from build123d import *

# Parameters (mm, degrees)
F0_W     = 75.805991888
F0_H     = 35.9990932047
F1_DEPTH = 25.4
F3_W     = 3.6910921335
F3_H     = 8.858628571
F3_W_2   = 4.4293105602
F3_H_2   = 7.0130825043
F4_DEPTH = 25.4
F5_DEPTH = 25.4
F6_W     = 26.3966843486
F6_H     = 116.8616563082
F7_DEPTH = 25.4
F8_W     = 123.443312943
F8_H     = 25.7022343576
F9_DEPTH = 25.4


with BuildPart() as f1:
    # F0 (on Front) → F1 (new body)
    with BuildSketch(Plane.XZ):
        with Locations((-37.902995944, 57.8962471336)):
            Rectangle(F0_W, F0_H)
    extrude(amount=F1_DEPTH)

    # F3 (on Front) → F4 (join)
    with BuildSketch(Plane.XZ):
        Polygon((-60.510866344, 33.7904244661), (-54.6051189303, 33.7904244661), (-54.6051189303, 33.0522060394), (-60.510866344, 33.0522060394), (-60.510866344, 29.3611101806), (-52.3904636502, 29.3611101806), (-52.3904636502, 38.2197387516), (-60.510866344, 38.2197387516), align=None)
        Polygon((-60.510866344, 33.0522060394), (-60.510866344, 33.7904244661), (-60.510866344, 38.2197387516), (-52.3904636502, 38.2197387516), (-52.3904636502, 59.6280917525), (-75.2752497792, 59.6280917525), (-75.2752497792, -67.7146911621), (-70.845939219, -67.7146911621), (-70.845939219, -74.7277736664), (-52.3904636502, -74.7277736664), (-52.3904636502, 29.3611101806), (-60.510866344, 29.3611101806), align=None)
        with Locations((-50.5449175835, 33.7904244661)):
            Rectangle(F3_W, F3_H)
        with Locations((-73.0605944991, -71.2212324142)):
            Rectangle(F3_W_2, F3_H_2)
        Polygon((-70.845939219, -81.7408561707), (-70.845939219, -74.7277736664), (-75.2752497792, -74.7277736664), (-75.2752497792, -67.7146911621), (-79.7045603395, -67.7146911621), (-79.7045603395, -81.7408561707), align=None)
    extrude(amount=F4_DEPTH)

    # F2 (on Front) → F5 (join)
    with BuildSketch(Plane.XZ):
        Polygon((74.952326715, 40.4343977571), (74.952326715, 75.4998028278), (0, 75.4998028278), (0, 40.4343977571), (25.4916474223, 40.4343977571), align=None)
    extrude(amount=F5_DEPTH)

    # F6 (on Front) → F7 (join)
    with BuildSketch(Plane.XZ):
        with Locations((61.6374202073, -17.1837881207)):
            Rectangle(F6_W, F6_H)
    extrude(amount=F7_DEPTH)

    # F8 (on Front) → F9 (join)
    with BuildSketch(Plane.XZ):
        with Locations((-13.6707611382, -62.0693061501)):
            Rectangle(F8_W, F8_H)
    extrude(amount=F9_DEPTH)


solid = f1.part
Verification items for the finished model (mm, model axes). A direction names the side the tool comes from. Coordinates: 2 decimals unless noted, no trailing zeros. Loops run counter-clockwise (first coordinate to the right, second up) from the corner with the lowest first, then second, coordinate; pieces in that order, holes last. Notation, with made-up numbers: (48.5, -21) -> (53.5, -21) arc R27 ccw to (53.5, 15) -> close; hole circle Ø6 at (47, 47.25). An arc over 180 degrees is marked (long way). Answer as CSV lines item,"result".
1) Depth check by flat-ended pin: pin 1 (1 mm diameter, centred on x = 11, z = -47.5, fed in from +Y); pin 2 (8 mm diameter, centred on x = 46.5, y = -3, fed in from +Z); pin 3 (6 mm diameter, centred on y = -10.5, z = 1, fed in from +X); pin 4 (2 mm diameter, centred on x = -78.5, y = -17.5, fed in from +Z). Enter the tip coordinate at first touch or a pass-through.
Found:
pin 1,"passes through"
pin 2,"stops at z = 75.5"
pin 3,"stops at x = 74.84"
pin 4,"stops at z = -67.71"
2) Thickness scan on L1, parallel to X at y = -17, z = -9; L2, parallel to X at y = -6.25, z = -69.5; L3, parallel to Z at x = -9.5, y = -15.75. Record the ranges inside material, lowest first. Write a range as from..to.
Found:
L1,"x = -75.28..-52.39, 48.44..74.84"
L2,"x = -79.7..48.05, 48.44..74.84"
L3,"z = -74.92..-49.22, 39.9..75.9"
3) Release check for a two-part mould opening along Z. For faces 1 (the flat face through (-75, -13, -81.741)), 2 (the flat face through (-58, -13, 33.052)), 3 (the flat face through (-55, -25.4, -2)), 4 (the flat face through (38, -13, 75.5)) record: +Z half, -Z half, draft (parallel to the pull), parting line (faces both ways), or undercut.
Found:
face 1,"-Z half"
face 2,"undercut"
face 3,"draft"
face 4,"+Z half"
4) Cross-section at D-D, the plane x = 55. Record the cut outline in (y, z), then the cut area to 3 significant figures.
Found:
outline,"(-25.4, -75.61) -> (0, -75.61) -> (0, 75.5) -> (-25.4, 75.5) -> close"
area,"3,840 mm2"
5) Tool access check on faces 5 (the flat face through (-75.392, -13, -59)), 6 (the flat face through (-52.39, -13, -10)), 7 (the flat face through (48.439, -13, -18)). Record the directions out of +Z, -Z, +X, -X, +Y, -Y that give a thin tool (end or side, any length) a straight path to the whole face; none if there is none.
Found:
face 5,"-X, +Y, -Y"
face 6,"+Y, -Y"
face 7,"-Z, +Y, -Y"
6) Cross-section at C-C, the plane z = 6. Record the cut outline in (x, y), then the cut area to 3 significant figures.
Found:
outline,"(-75.28, -25.4) -> (-52.39, -25.4) -> (-52.39, 0) -> (-75.28, 0) -> close; (48.44, -25.4) -> (74.84, -25.4) -> (74.84, 0) -> (48.44, 0) -> close"
area,"1,250 mm2"
7) Cross-section at A-A, the plane x = 17.5. Record the cut outline in (y, z), then the cut area to 3 significant figures.
Found:
outline,"(-25.4, -74.92) -> (0, -74.92) -> (0, -49.22) -> (-25.4, -49.22) -> close; (-25.4, 40.43) -> (0, 40.43) -> (0, 75.5) -> (-25.4, 75.5) -> close"
area,"1,540 mm2"
